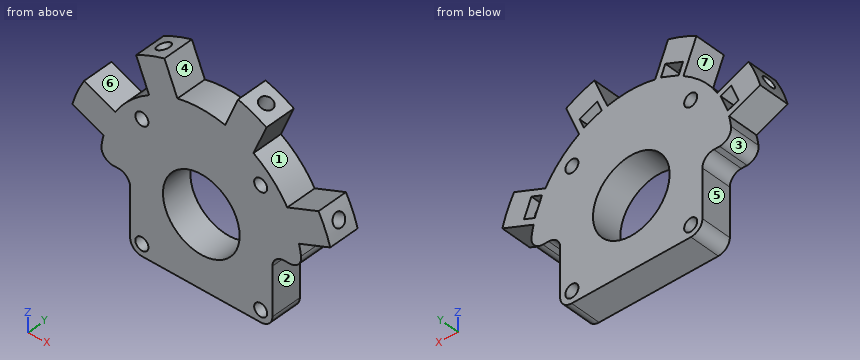
from build123d import *

# Parameters (mm, degrees)
SALIENTE_EXTRUIR1_DEPTH = 8
CROQUIS3_R              = 1.7
CORTAR_EXTRUIR1_DEPTH   = 10
CORTAR_EXTRUIR2_DEPTH   = 7
MATRIZC1_COUNT          = 4
MATRIZC1_ANGLE          = 135
CROQUIS5_R              = 10
CROQUIS5_R_2            = 1.7
CORTAR_EXTRUIR3_DEPTH   = 8
CORTAR_EXTRUIR4_DEPTH   = 8
REDONDEO1_R             = 3


with BuildPart() as part:
    # Croquis1 → Saliente-Extruir1 (new body)
    with BuildSketch(Plane(origin=(0, 0, 0), x_dir=(1, 0, 0), z_dir=(0, 1, 0))):
        with BuildLine():
            Line((-33.65465082, -9.610644005), (-25.499354444, -6.232609641))
            ThreePointArc((-25.499354444, -6.232609641), (0, 26.25), (25.499354444, -6.232609641))
            Line((25.499354444, -6.232609641), (33.65465082, -9.610644005))
            ThreePointArc((33.65465082, -9.610644005), (32.335783638, -13.393920133), (30.593183361, -17.001680265))
            Line((30.593183361, -17.001680265), (22.437886985, -13.623645901))
            ThreePointArc((22.437886985, -13.623645901), (18.561553006, -18.561553006), (13.623645901, -22.437886985))
            Line((13.623645901, -22.437886985), (17.001680265, -30.593183361))
            ThreePointArc((17.001680265, -30.593183361), (13.393920133, -32.335783638), (9.610644005, -33.65465082))
            Line((9.610644005, -33.65465082), (6.232609641, -25.499354444))
            ThreePointArc((6.232609641, -25.499354444), (0, -26.25), (-6.232609641, -25.499354444))
            Line((-6.232609641, -25.499354444), (-9.610644005, -33.65465082))
            ThreePointArc((-9.610644005, -33.65465082), (-13.393920133, -32.335783638), (-17.001680265, -30.593183361))
            Line((-17.001680265, -30.593183361), (-13.623645901, -22.437886985))
            ThreePointArc((-13.623645901, -22.437886985), (-18.561553006, -18.561553006), (-22.437886985, -13.623645901))
            Line((-22.437886985, -13.623645901), (-30.593183361, -17.001680265))
            ThreePointArc((-30.593183361, -17.001680265), (-32.335783638, -13.393920133), (-33.65465082, -9.610644005))
        make_face()
    extrude(amount=SALIENTE_EXTRUIR1_DEPTH)

    # Croquis3 → Cortar-Extruir1 (cut)
    with BuildSketch(Plane(origin=(-32.335783638, 0, 13.393920133), x_dir=(0.382683432, 0, 0.923879533), z_dir=(-0.923879533, 0, 0.382683432))):
        with Locations((0, 4)):
            Circle(CROQUIS3_R)
    cortar_extruir1 = extrude(amount=-CORTAR_EXTRUIR1_DEPTH, mode=Mode.SUBTRACT)

    # Croquis4 → Cortar-Extruir2 (cut)
    with BuildSketch(Plane(origin=(0, 8, 0), x_dir=(1, 0, 0), z_dir=(0, 1, 0))):
        Polygon((-27.980184907, -8.883791565), (-26.066767745, -13.503189228), (-23.295129148, -12.355138931), (-25.208546309, -7.735741268), align=None)
    cortar_extruir2 = extrude(amount=-CORTAR_EXTRUIR2_DEPTH, mode=Mode.SUBTRACT)

    # MatrizC1: Cortar-Extruir1, Cortar-Extruir2 ×4 about axis
    matrizc1_axis = Axis((0, 0, 0), (0, 1, 0))
    for i in range(1, MATRIZC1_COUNT):
        add(cortar_extruir1.rotate(matrizc1_axis, i * MATRIZC1_ANGLE / (MATRIZC1_COUNT - 1)), mode=Mode.SUBTRACT)
        add(cortar_extruir2.rotate(matrizc1_axis, i * MATRIZC1_ANGLE / (MATRIZC1_COUNT - 1)), mode=Mode.SUBTRACT)

    # Croquis5 → Cortar-Extruir3 (cut)
    with BuildSketch(Plane(origin=(0, 8, 0), x_dir=(1, 0, 0), z_dir=(0, 1, 0))):
        Circle(CROQUIS5_R)
        with Locations((-15.5, 15.5)):
            Circle(CROQUIS5_R_2)
        with Locations((15.5, 15.5)):
            Circle(CROQUIS5_R_2)
        with Locations((15.5, -15.5)):
            Circle(CROQUIS5_R_2)
        with Locations((-15.5, -15.5)):
            Circle(CROQUIS5_R_2)
    extrude(amount=-CORTAR_EXTRUIR3_DEPTH, mode=Mode.SUBTRACT)

    # Croquis6 → Cortar-Extruir4 (cut)
    with BuildSketch(Plane(origin=(0, 8, 0), x_dir=(1, 0, 0), z_dir=(0, 1, 0))):
        Polygon((18.561553006, 18.561553006), (-18.561553006, 18.561553006), (-18.561553006, 0), (-26.25, 0), (-26.25, 31.288102552), (26.25, 31.288102552), (26.25, 0), (18.561553006, 0), align=None)
    extrude(amount=-CORTAR_EXTRUIR4_DEPTH, mode=Mode.SUBTRACT)

    # Redondeo1
    redondeo1_edges = [part.edges().sort_by_distance(p)[0] for p in [
        (-18.561553006, 4, -18.561553006),
        (-18.561553006, 4, 0),
        (-26.25, 4, 0),
        (26.25, 4, 0),
        (18.561553006, 4, 0),
        (18.561553006, 4, -18.561553006),
    ]]
    fillet(redondeo1_edges, radius=REDONDEO1_R)


solid = part.part
Check sheet for the modelled part. Datum: model origin and axes. Units: mm. Face numbers are marked on the shaded views. A direction names the side the tool comes from. Give positions to 0.01 mm unless a question says otherwise; leave off trailing zeros. Order: outer loops, then holes, each group sorted by start corner. A loop starts at its lowest first (then second) coordinate and runs counter-clockwise, first axis right, second up. Notation, with made-up numbers: (86, 45) - (145, 45) arc R12 cw to (145, 57) - close; hole circle Ø11 at (37.5, 75). An arc over 180 degrees is marked (long way). Answer as CSV lines item,"result".
1. Go/stop test with flat-tipped pins: P1, Ø12, axis at x = 0, z = 0, coming from the -Y side; P2, Ø1, axis at y = 3, z = 7, coming from the +X side; P3, Ø0.7, axis at x = 22.5, y = 6, coming from the -Z side; P4, Ø2, axis at y = 4.5, z = 19, coming from the +X side. Record where each tip stops, or that it passes through.
Result sheet:
P1,"through"
P2,"x = 28.56"
P3,"z = 0"
P4,"x = 19.11"
2. Section check A-A (x = 0). Record the boundary of the cut face in (y, z).
Result sheet:
outline,"(0, -18.56) - (8, -18.56) - (8, -10) - (0, -10) - close; (0, 10) - (8, 10) - (8, 26.25) - (0, 26.25) - close"
3. Mould release check, pull along X, two halves, no side actions. Record for the marked faces 1, 2, 3 and 4: released by +X, released by -X, zero draft, split by the parting line, or undercut.
Result sheet:
face 1,"undercut"
face 2,"released by +X"
face 3,"released by -X"
face 4,"undercut"
4. Section check C-C (x = 20). Record the boundary of the cut face in (y, z), then the cut area to 3 significant figures.
Result sheet:
outline,"(0, -0.44) - (8, -0.44) - (8, 17) - (0, 17) - close"
area,"140 mm²"
5. Section check B-B (y = 3). State how many separate pieces and enclosed holes the cut face has, then the cut area to 3 significant figures.
Result sheet:
separate pieces,"1"
enclosed holes,"5"
area,"1,560 mm²"
6. Tool access check on the marked faces 5, 6 and 7. Record the directions out of +Z, -Z, +X, -X, +Y, -Y that give a thin tool (end or side, any length) a straight path to the whole face; none if there is none.
Result sheet:
face 5,"-Z, -X, +Y, -Y"
face 6,"+Z, +Y, -Y"
face 7,"-X, +Y, -Y"
7. Scan lines: probe 1 along X at (y, z) = (4.75, -15.5); probe 2 along Z at (x, y) = (8, 7.75); probe 3 along Z at (x, y) = (15, 3.5). Record each from-to range of solid material in increasing order. Write a range as from..to.
Result sheet:
probe 1,"-18.56..-17.2, -13.8..13.8, 17.2..18.56"
probe 2,"-18.56..-6, 6..25.1, 25.85..29.77"
probe 3,"-18.56..-17.12, -13.88..13.88, 17.12..21.54, 25.76..31.62"
